Input: part model. Units: mm. Frame: model coordinates. Face numbers are marked on the shaded views. A direction names the side the tool comes from. Coordinates: 2 decimals unless noted, no trailing zeros. Loops run counter-clockwise (first coordinate to the right, second up) from the corner with the lowest first, then second, coordinate; pieces in that order, holes last. Notation, with made-up numbers: (3, 3.5) - (36, 3.5) arc R29 ccw to (36, 42.5) - close; hole circle Ø2 at (8.25, 41). An arc over 180 degrees is marked (long way). Use a Markdown table: item, result. Add a question column.
1. Access query for the marked faces 1 and 2. Directions: +Z, -Z, +X, -X, +Y, -Y. A direction counts if a zero-diameter tool reaches every point of the face in a straight line with its end or side. Return the directions, or none.
2. Contact query for a flat-ended pin moving along its axis: P1, Ø2, axis at y = 0.5, z = -8, coming from the +X side. Output: stop coordinate, or through.
3. Draft query along X for the marked faces 3 and 4. Return one class per face: released by +X, released by -X, zero draft, split by the parting line, or undercut.
4. Section query C-C on x = -3.25. Return the cut outline in (y, z).
5. Ray query, L1, parallel to Y at x = -2, z = -1.75; L2, parallel to Y at x = -2.75, z = -5; L3, parallel to Y at x = 0.5, z = -3.5. Return the intervals inside material, ascending. Write a range as [from, to].
6. Section query A-A on x = 1. Return the cut outline in (y, z), then the cut area to 3 significant figures.
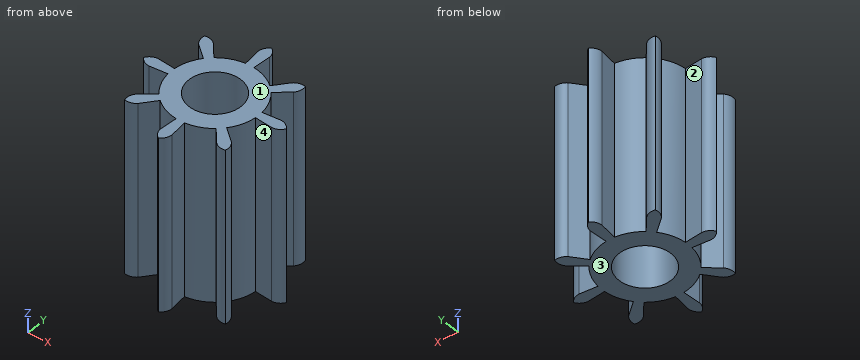
```python
from build123d import *

# Parameters (mm, degrees)
SKETCH1_R           = 1.5
BOSS_EXTRUDE1_DEPTH = 10
CIRPATTERN1_COUNT   = 8


with BuildPart() as part:
    # Sketch1 → Boss-Extrude1 (new body)
    with BuildSketch(Plane.XY):
        with BuildLine():
            Line((-0.33, 3.484408128), (-0.235714286, 2.488862948))
            ThreePointArc((-0.235714286, 2.488862948), (0, -2.5), (0.235714286, 2.488862948))
            Line((0.235714286, 2.488862948), (0.33, 3.484408128))
            ThreePointArc((0.33, 3.484408128), (0.241576766, 3.814408128), (0, 4.055984894))
            ThreePointArc((0, 4.055984894), (-0.241576766, 3.814408128), (-0.33, 3.484408128))
        make_face()
        Circle(SKETCH1_R, mode=Mode.SUBTRACT)
    boss_extrude1 = extrude(amount=-BOSS_EXTRUDE1_DEPTH)

    # CirPattern1: Boss-Extrude1 ×8 about axis
    cirpattern1_axis = Axis((0, 0, 0), (0, 0, 1))
    for i in range(1, CIRPATTERN1_COUNT):
        add(boss_extrude1.rotate(cirpattern1_axis, i * 360 / CIRPATTERN1_COUNT))


solid = part.part
```
Resolved:
| question | item | result |
|---|---|---|
| 1 | face 1 | +Z, +X, -X, +Y, -Y |
| 1 | face 2 | +Z, -Z |
| 2 | P1 | x = 4.06 |
| 3 | face 3 | zero draft |
| 3 | face 4 | undercut |
| 4 | outline | (-0.31, -10) - (0.31, -10) - (0.31, 0) - (-0.31, 0) - close |
| 5 | L1 | [-2.42, -1.65], [-1.5, 1.5], [1.65, 2.42] |
| 5 | L2 | [-2.89, -2.29], [-0.26, 0.26], [2.29, 2.89] |
| 5 | L3 | [-2.45, -1.41], [1.41, 2.45] |
| 6 | outline | (-2.29, -10) - (-1.12, -10) - (-1.12, 0) - (-2.29, 0) - close; (1.12, -10) - (2.29, -10) - (2.29, 0) - (1.12, 0) - close |
| 6 | area | 23.5 mm² |
